Geometry check sheet. Reference: the model listing, model coordinates, mm. Face numbers are marked on the shaded views. A direction names the side the tool comes from. Give positions to 0.01 mm unless a question says otherwise; leave off trailing zeros. Order: outer loops, then holes, each group sorted by start corner. A loop starts at its lowest first (then second) coordinate and runs counter-clockwise, first axis right, second up.
from build123d import *

# Parameters (mm, degrees)
BOSS_EXTRUDE1_DEPTH = 9
CUT_EXTRUDE1_REACH  = 20
SKETCH3_R           = 2.38125
CUT_EXTRUDE2_REACH  = 3.5
SKETCH4_R           = 1.75
FILLET1_R           = 1
FILLET2_R           = 1


with BuildPart() as part:
    # Sketch1 → Boss-Extrude1 (new body, symmetric)
    with BuildSketch(Plane.XY):
        with BuildLine():
            Line((-10, 0), (-4, 0))
            ThreePointArc((-4, 0), (-3.92634671, 0.76406905), (-3.708099244, 1.5))
            Line((-3.708099244, 1.5), (-10, 1.5))
            Line((-10, 1.5), (-10, 0))
        make_face()
        with BuildLine():
            Line((-4, 0), (4, 0))
            ThreePointArc((4, 0), (3.92634671, 0.76406905), (3.708099244, 1.5))
            Line((3.708099244, 1.5), (-3.708099244, 1.5))
            ThreePointArc((-3.708099244, 1.5), (-3.92634671, 0.76406905), (-4, 0))
        make_face()
        with BuildLine():
            ThreePointArc((3.708099244, 1.5), (3.92634671, 0.76406905), (4, 0))
            Line((4, 0), (10, 0))
            Line((10, 0), (10, 1.5))
            Line((10, 1.5), (3.708099244, 1.5))
        make_face()
        with BuildLine():
            Line((-3.708099244, 1.5), (3.708099244, 1.5))
            ThreePointArc((3.708099244, 1.5), (0, 4), (-3.708099244, 1.5))
        make_face()
    extrude(amount=BOSS_EXTRUDE1_DEPTH, both=True)

    # Sketch3 → Cut-Extrude1 (cut, up to next)
    with BuildSketch(Plane.XY.offset(9), mode=Mode.PRIVATE) as cut_extrude1_sk1:
        with Locations((0, -0.5)):
            Circle(SKETCH3_R)
    cut_extrude1_tool1 = extrude(cut_extrude1_sk1.sketch, amount=-CUT_EXTRUDE1_REACH, mode=Mode.PRIVATE) & part.part
    add(cut_extrude1_tool1.solids().sort_by_distance((0, -0.5, 9))[0], mode=Mode.SUBTRACT)

    # Sketch4 → Cut-Extrude2 (cut, up to next)
    with BuildSketch(Plane(origin=(0, 1.5, 0), x_dir=(1, 0, 0), z_dir=(0, 1, 0)), mode=Mode.PRIVATE) as cut_extrude2_sk1:
        with Locations((-6.8, 5)):
            Circle(SKETCH4_R)
    cut_extrude2_tool1 = extrude(cut_extrude2_sk1.sketch, amount=-CUT_EXTRUDE2_REACH, mode=Mode.PRIVATE) & part.part
    add(cut_extrude2_tool1.solids().sort_by_distance((-6.8, 1.5, -5))[0], mode=Mode.SUBTRACT)
    # Sketch4 → Cut-Extrude2 (cut, up to next)
    with BuildSketch(Plane(origin=(0, 1.5, 0), x_dir=(1, 0, 0), z_dir=(0, 1, 0)), mode=Mode.PRIVATE) as cut_extrude2_sk2:
        with Locations((6.8, 5)):
            Circle(SKETCH4_R)
    cut_extrude2_tool2 = extrude(cut_extrude2_sk2.sketch, amount=-CUT_EXTRUDE2_REACH, mode=Mode.PRIVATE) & part.part
    add(cut_extrude2_tool2.solids().sort_by_distance((6.8, 1.5, -5))[0], mode=Mode.SUBTRACT)
    # Sketch4 → Cut-Extrude2 (cut, up to next)
    with BuildSketch(Plane(origin=(0, 1.5, 0), x_dir=(1, 0, 0), z_dir=(0, 1, 0)), mode=Mode.PRIVATE) as cut_extrude2_sk3:
        with Locations((6.8, -5)):
            Circle(SKETCH4_R)
    cut_extrude2_tool3 = extrude(cut_extrude2_sk3.sketch, amount=-CUT_EXTRUDE2_REACH, mode=Mode.PRIVATE) & part.part
    add(cut_extrude2_tool3.solids().sort_by_distance((6.8, 1.5, 5))[0], mode=Mode.SUBTRACT)
    # Sketch4 → Cut-Extrude2 (cut, up to next)
    with BuildSketch(Plane(origin=(0, 1.5, 0), x_dir=(1, 0, 0), z_dir=(0, 1, 0)), mode=Mode.PRIVATE) as cut_extrude2_sk4:
        with Locations((-6.8, -5)):
            Circle(SKETCH4_R)
    cut_extrude2_tool4 = extrude(cut_extrude2_sk4.sketch, amount=-CUT_EXTRUDE2_REACH, mode=Mode.PRIVATE) & part.part
    add(cut_extrude2_tool4.solids().sort_by_distance((-6.8, 1.5, 5))[0], mode=Mode.SUBTRACT)

    # Fillet1
    fillet1_edges = [part.edges().sort_by_distance(p)[0] for p in [
        (10, 0.75, -9),
        (-10, 0.75, -9),
        (-10, 0.75, 9),
        (10, 0.75, 9),
    ]]
    fillet(fillet1_edges, radius=FILLET1_R)

    # Fillet2
    fillet2_edges = [part.edges().sort_by_distance(p)[0] for p in [
        (-3.708099244, 1.5, 0),
        (3.708099244, 1.5, 0),
    ]]
    fillet(fillet2_edges, radius=FILLET2_R)


solid = part.part
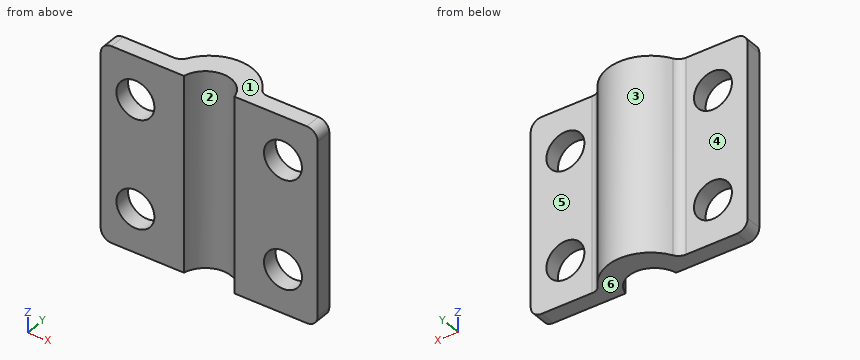
Item 1: Sectioned sample at C-C (z = 5). Enter the section's corners in (x, y).
Reported:
outline: (-10, 0) - (-8.55, 0) - (-8.55, 1.5) - (-10, 1.5) - close; (-5.05, 0) - (-2.33, 0) arc R2.38 cw to (2.33, 0) - (5.05, 0) - (5.05, 1.5) - (4.33, 1.5) arc R1 cw to (3.46, 2) arc R4 ccw to (-3.46, 2) arc R1 cw to (-4.33, 1.5) - (-5.05, 1.5) - close; (8.55, 0) - (10, 0) - (10, 1.5) - (8.55, 1.5) - close
Item 2: Sectioned sample at B-B (x = -6.8). Enter the section's corners in (y, z).
Reported:
outline: (0, -9) - (1.5, -9) - (1.5, -6.75) - (0, -6.75) - close; (0, -3.25) - (1.5, -3.25) - (1.5, 3.25) - (0, 3.25) - close; (0, 6.75) - (1.5, 6.75) - (1.5, 9) - (0, 9) - close
Item 3: Gauge pin test, flat ends, axial feed: pin 1 (1.7 mm diameter, centred on x = 7, z = -3.5, fed in from +Y); pin 2 (3 mm diameter, centred on x = 6.8, z = 5, fed in from +Y); pin 3 (1 mm diameter, centred on y = 2.5, z = -3, fed in from -X). Record the tip position at first contact, or that the pin passes through.
Reported:
pin 1: stops at y = 1.5
pin 2: passes through
pin 3: stops at x = -3.46
Item 4: Scan lines: L1, parallel to Z at x = 6.8, y = 0.9; L2, parallel to X at y = 0.65, z = 5.5; L3, parallel to X at y = 1.15, z = 5. Record each from-to range of solid material in increasing order.
Reported:
L1: z = -9 to -6.75, -3.25 to 3.25, 6.75 to 9
L2: x = -10 to -8.48, -5.12 to -2.09, 2.09 to 5.12, 8.48 to 10
L3: x = -10 to -8.55, -5.05 to -1.72, 1.72 to 5.05, 8.55 to 10
Item 5: Set-up check for the marked faces 4, 5 and 6: record each of +Z, -Z, +X, -X, +Y, -Y from which the full face is reachable in a straight line by a thin tool's end or side.
Reported:
face 4: +Z, -Z, -X, +Y
face 5: +Z, -Z, +X, +Y
face 6: -Z, +X, -X, +Y, -Y
Item 6: Draft check along X on the marked faces 1, 2 and 3. Enter one of: released by +X, released by -X, zero draft, split by the parting line, or undercut.
Reported:
face 1: zero draft
face 2: undercut
face 3: split by the parting line
Item 7: Sectioned sample at D-D (z = 1). Enter the section's corners in (x, y).
Reported:
outline: (-10, 0) - (-2.33, 0) arc R2.38 cw to (2.33, 0) - (10, 0) - (10, 1.5) - (4.33, 1.5) arc R1 cw to (3.46, 2) arc R4 ccw to (-3.46, 2) arc R1 cw to (-4.33, 1.5) - (-10, 1.5) - close
Item 8: Sectioned sample at A-A (y = 0.75). Enter the section's corners in (x, z).
Reported:
outline: (-10, -8) arc R1 ccw to (-9, -9) - (-2.03, -9) - (-2.03, 9) - (-9, 9) arc R1 ccw to (-10, 8) - close; (2.03, -9) - (9, -9) arc R1 ccw to (10, -8) - (10, 8) arc R1 ccw to (9, 9) - (2.03, 9) - close; hole circle Ø3.5 at (-6.8, -5); hole circle Ø3.5 at (-6.8, 5); hole circle Ø3.5 at (6.8, -5); hole circle Ø3.5 at (6.8, 5)
